Autodesk Inventor part; units mm, degrees
ref_plane "YZ Plane" through (0, 0, 0) normal (1, 0, 0) x (0, 1, 0)
ref_plane "XZ Plane" through (0, 0, 0) normal (0, 1, 0) x (-1, 0, 0)
ref_plane "XY Plane" through (0, 0, 0) normal (0, 0, 1) x (1, 0, 0)
sketch "Sketch1" plane through (0, 0, 0) normal (0, 0, 1) x (1, 0, 0)
  line L0 (0, 0) -> (14, 0)
  line L1 (14, 0) -> (14, -14)
  line L2 (14, -14) -> (0, -14)
  line L3 (0, -14) -> (0, 0)
  dimension "d0" = 14
  dimension "d1" = 14
extrude "Extrusion1" add sketch "Sketch1" against normal blind 22
sketch "Sketch2" plane through (0, 0, 0) normal (0, 0, 1) x (1, 0, 0)
  line L0 (2, -2) -> (12, -2)
  line L1 (12, -2) -> (12, -22)
  line L2 (12, -22) -> (2, -22)
  line L3 (2, -22) -> (2, -2)
  point P0 (0, 0)
  dimension "d4" = 10
  dimension "d5" = 20
extrude "Extrusion2" cut sketch "Sketch2" against normal blind 20
sketch "Sketch8" plane through (0, -14, 0) normal (-1, 0, 0) x (0, 0, 1)
  point P0 (0, 14)
sketch "Sketch9" plane through (0, -14, 0) normal (-1, 0, 0) x (0, 0, 1)
  point P0 (0, 14)
sketch "Sketch11" plane through (0, -14, 0) normal (-1, 0, 0) x (0, 0, 1)
  point P0 (0, 14)
sketch "Sketch14" plane through (0, -14, 0) normal (-1, 0, 0) x (0, 0, 1)
  point P0 (0, 14)
sketch "Sketch15" plane through (0, -14, 0) normal (-1, 0, 0) x (0, 0, 1)
  point P0 (0, 14)
sketch "Sketch16" plane through (0, -14, 0) normal (-1, 0, 0) x (0, 0, 1)
  line L0 (-12.5, 12) -> (-17.5, 12)
  line L1 (-17.5, 12) -> (-17.5, 0)
  line L2 (-17.5, 0) -> (-12.5, 0)
  line L3 (-12.5, 0) -> (-12.5, 12)
  point P0 (0, 14)
  dimension "d30" = 5
  dimension "d31" = 12
extrude "Extrusion10" cut sketch "Sketch16" against normal blind 2
sketch "Sketch17" plane through (0, 0, -20) normal (0, 0, 1) x (1, 0, 0)
  line L0 (12, -2) -> (7.5, -2)
  line L1 (7.5, -2) -> (7.5, -6.5)
  line L2 (7.5, -6.5) -> (12, -6.5)
  line L3 (12, -6.5) -> (12, -2)
  point P0 (0, 0)
  dimension "d34" = 4.5
  dimension "d35" = 4.5
extrude "Extrusion11" add sketch "Sketch17" along normal blind 9
fillet "Fillet1" radius 0.8 8 edges at (0, -8, -12.5) (2, -8, -12.5) (0, -2, -15) (0, -8, -17.5) (2, -8, -17.5) (12, -14, -10) (7.5, -6.5, -15.5) (9.75, -6.5, -11)
properties part number "housing_v07"
For this review, take the finished solid that the model builds, in its own axes (mm). A direction names the side the tool comes from. Coordinates: 2 decimals unless noted, no trailing zeros. Write each loop counter-clockwise with the first axis right and the second up, starting at its lowest first coordinate (ties: lowest second). Pieces come first, ordered by that corner, then holes.
(1) The part is to be moulded in two halves that separate along X. For faces 5 (the face through (0.24, -1.77, -15.05)), 6 (the face through (6, -2, -8)), 7 (the face through (6.4, -1.8, 0)), 8 (the face through (14, -7, -11)), say which applies: +X half, -X half, draft (parallel to the pull), parting line (faces both ways), or undercut.
(2) Add section A-A on y = -3.5. Give the boundary of the cut face in (x, z), then the cut area to 3 significant figures.
(3) For pin 1 Ø1.5 at (x, z) = (8.5, -12.5) entering from -Y; pin 2 Ø3.5 at (x, z) = (9, -9.5) entering from -Y; pin 3 Ø1.1 at (x, y) = (9.5, -4) entering from +Z, all flat-tipped, find the tip position at first contact; note any pin that passes through.
(4) Add section C-C on z = -14.25. Give the boundary of the cut face in (x, y), then the cut area to 3 significant figures.
(5) Add section B-B on x = 3.5. Give the boundary of the cut face in (y, z).
(6) Wall thickness on probe 1 along X at (y, z) = (-5, -10); probe 2 along Z at (x, y) = (1, -7); probe 3 along Z at (x, y) = (6.5, -9.5): over which ranges is each line inside the solid? List them lowest first.
(7) Tool access review of faces 1 (the face through (1.77, -7.92, -12.26)), 2 (the face through (2, -8, -6)), 3 (the face through (0.24, -7.51, -12.27)), 4 (the face through (0, -7, -8)): name each direction out of +Z, -Z, +X, -X, +Y, -Y from which nothing blocks a thin tool from reaching the whole face with its end or side.
(8) Add section D-D on y = -10.5. Give the boundary of the cut face in (x, z).
Answer sheet:
1. face 5: -X half
1. face 6: undercut
1. face 7: draft
1. face 8: +X half
2. outline: (0, -22) - (14, -22) - (14, 0) - (12, 0) - (12, -11) - (7.5, -11) - (7.5, -20) - (2, -20) - (2, -18.3) arc R0.8 ccw to (1.2, -17.5) - (0.8, -17.5) arc R0.8 ccw to (0, -18.3) - close; (0, -11.7) arc R0.8 ccw to (0.8, -12.5) - (1.2, -12.5) arc R0.8 ccw to (2, -11.7) - (2, 0) - (0, 0) - close
2. area: 138 mm2
3. pin 1: stops at y = -6.5
3. pin 2: stops at y = -6.28
3. pin 3: stops at z = -11
4. outline: (0, -1.2) arc R0.8 ccw to (0.8, -2) - (7.5, -2) - (7.5, -5.7) arc R0.8 ccw to (8.3, -6.5) - (12, -6.5) - (12, -13.2) arc R0.8 ccw to (12.8, -14) - (14, -14) - (14, 0) - (0, 0) - close
4. area: 71.8 mm2
5. outline: (-14, -22) - (0, -22) - (0, 0) - (-2, 0) - (-2, -20) - (-14, -20) - close
6. probe 1: x = 0 to 2, 12 to 14
6. probe 2: z = -22 to -17.5, -12.5 to 0
6. probe 3: z = -22 to -20
7. face 1: -Y
7. face 2: +Z, -Y
7. face 3: -X, -Y
7. face 4: +Z, -Z, -X, +Y, -Y
8. outline: (0, -22) - (14, -22) - (14, 0) - (12, 0) - (12, -20) - (2, -20) - (2, -18.3) arc R0.8 ccw to (1.2, -17.5) - (0.8, -17.5) arc R0.8 ccw to (0, -18.3) - close; (0, -11.7) arc R0.8 ccw to (0.8, -12.5) - (1.2, -12.5) arc R0.8 ccw to (2, -11.7) - (2, 0) - (0, 0) - close
